Autodesk Inventor part; units mm, degrees
ref_plane "YZ Plane" through (0, 0, 0) normal (1, 0, 0) x (0, 1, 0)
ref_plane "XZ Plane" through (0, 0, 0) normal (0, 1, 0) x (-1, 0, 0)
ref_plane "XY Plane" through (0, 0, 0) normal (0, 0, 1) x (1, 0, 0)
sketch "Sketch1" plane through (0, 0, 0) normal (0, 0, 1) x (1, 0, 0)
  line L0 (4.5, -4.5) -> (-4.5, -4.5)
  line L1 (-4.5, -4.5) -> (-4.5, 4.5)
  line L2 (-4.5, 4.5) -> (4.5, 4.5)
  line L3 (4.5, 4.5) -> (4.5, -4.5)
  line L4 (4.5, -4.5) -> (-4.5, 4.5) construction
  line L5 (-4.5, -4.5) -> (4.5, 4.5) construction
  point P0 (0, 0)
  dimension "d0" = 9
  dimension "d1" = 9
extrude "Extrusion1" add sketch "Sketch1" along normal blind 2
sketch "Sketch2" plane through (0, 0, 2) normal (0, 0, 1) x (1, 0, 0)
  line L0 (-4.5, -4.5) -> (4.5, -4.5)
  line L1 (4.5, -4.5) -> (4.5, 4.5)
  line L2 (4.5, 4.5) -> (-4.5, 4.5)
  line L3 (-4.5, 4.5) -> (-4.5, -4.5)
  circle A0 centre (0, 0) radius 4.2
  circle A1 centre (0, 0) radius 3.5
  dimension "d4" = 8.4
  dimension "d5" = 7
extrude "Extrusion2" add sketch "Sketch2" along normal blind 2 contours A0
properties part number "00_ESP32_Camera_only"
Design review of the part built by this model. Coordinates are the model's own, in mm. A direction names the side the tool comes from. Coordinates: 2 decimals unless noted, no trailing zeros. Loops run counter-clockwise (first coordinate to the right, second up) from the corner with the lowest first, then second, coordinate; pieces in that order, holes last. Notation, with made-up numbers: (40, 20) -> (61, 20) arc R25 cw to (61, 36) -> close; hole circle Ø7 at (54.5, 6.5). An arc over 180 degrees is marked (long way). Use a Markdown table: item, result. Add a question column.
Item 1: We need section C-C, the plane z = 2.95. Write out the cut boundary in (x, y).
Item 2: The part is to be moulded in two halves that separate along Y. For faces 3 (the cylindrical face through (3.233, 1.341, 2.986)), 4 (the flat face through (-4.5, 0, 1)), 5 (the cylindrical face through (4.006, -1.262, 2.986)), 6 (the flat face through (0, 0, 2)), say which applies: +Y half, -Y half, draft (parallel to the pull), parting line (faces both ways), or undercut.
Item 3: Wall thickness on L1, parallel to Y at x = 0, z = 2.7; L2, parallel to Z at x = -1.5, y = -2.75; L3, parallel to Y at x = 3, z = 3.3: over which ranges is each line inside the solid? List them lowest first. Write a range as from..to.
Item 4: Machinability: for faces 1 (the flat face through (0, 0, 0)), 2 (the flat face through (-4, 2, 2)), which of the approach directions +Z, -Z, +X, -X, +Y, -Y give a long, thin tool a straight path to every point of the face, cutting with its end or side? Answer none if there is none.
Item 5: We need section A-A, the plane x = 0. Write out the cut boundary in (y, z).
Item 6: Clearance check with a flat-ended pin moving along its axis: P1, Ø1, axis at x = -3.5, y = 2, coming from the -Z side. State where the tip first meets the part, or that it passes through.
Numbers:
| question | item | result |
|---|---|---|
| 1 | outline | circle Ø8.4 at (0, 0); hole circle Ø7 at (0, 0) |
| 2 | face 3 | undercut |
| 2 | face 4 | draft |
| 2 | face 5 | parting line |
| 2 | face 6 | undercut |
| 3 | L1 | y = -4.2..-3.5, 3.5..4.2 |
| 3 | L2 | z = 0..2 |
| 3 | L3 | y = -2.94..-1.8, 1.8..2.94 |
| 4 | face 1 | -Z, +X, -X, +Y, -Y |
| 4 | face 2 | +Z |
| 5 | outline | (-4.5, 0) -> (4.5, 0) -> (4.5, 2) -> (4.2, 2) -> (4.2, 4) -> (3.5, 4) -> (3.5, 2) -> (-3.5, 2) -> (-3.5, 4) -> (-4.2, 4) -> (-4.2, 2) -> (-4.5, 2) -> close |
| 6 | P1 | stops at z = 0 |
